Design review of the part built by this model. Coordinates are the model's own, in mm. A direction names the side the tool comes from. Coordinates: 2 decimals unless noted, no trailing zeros. Loops run counter-clockwise (first coordinate to the right, second up) from the corner with the lowest first, then second, coordinate; pieces in that order, holes last. Notation, with made-up numbers: M -29,65.5 L -8,65.5 A15 ccw -8,79.5 Z; hole C 84,85 d11. An arc over 180 degrees is marked long. Answer as a JSON object with one key per item and string values. Group by question number.
1. Consider section A-A (z = 8.5). Count the separate pieces of the cut face and the enclosed holes in it, then the cut area to 3 significant figures.
2. Draft analysis for pull direction Y (two halves, no side actions). For faces 1 (the flat face through (-1, 0, 7)), 2 (the cylindrical face through (36.41, -58.99, 6.9)), 3 (the cylindrical face through (58.975, -52.273, 6.902)), 4 (the flat face through (125, -35, 7)), state which applies: +Y half, -Y half, draft (parallel to the pull), parting line (faces both ways), or undercut.
3. Consider section C-C (x = -22.5). State the section outline as (y, z) points, then the cut area to 3 significant figures.
4. Insertion check: pin 1 (7 mm diameter, centred on x = 34.33, y = -55, fed in from +Z); pin 2 (4 mm diameter, centred on x = -18, z = 5.5, fed in from +Y). Each pin has a flat end and moves straight along its axis. Give the tip position at first contact, or say it passes through.
5. Machinability: for faces 5 (the flat face through (-110, 0, 7)), 6 (the flat face through (-2, -27, 0)), 7 (the flat face through (110, 0, 7)), which of the approach directions +Z, -Z, +X, -X, +Y, -Y give a long, thin tool a straight path to every point of the face, cutting with its end or side? Answer none if there is none.
6. Consider section B-B (x = -97.5). State the section outline as (y, z) points.
7. To check wall thickness, follow probe 1 along Y at (x, z) = (46, 8.75); probe 2 along Y at (x, z) = (12.5, 8.5); probe 3 along X at (y, z) = (-57.5, 3) (3 decimals). State the ranges of each line that lie inside material, in increasing order.
from build123d import *

# Parameters (mm, degrees)
F0_W     = 250
F0_H     = 70
F0_R     = 1.75
F0_R_2   = 5.75
F0_R_3   = 4.5
F0_R_4   = 3.5
F0_R_5   = 2.75
F0_R_6   = 2.25
F0_R_7   = 1.5
F0_R_8   = 1.25
F0_R_9   = 1
F0_R_10  = 3.75
F0_R_11  = 3.25
F0_R_12  = 3
F0_R_13  = 2.5
F0_R_14  = 2
F1_DEPTH = 14
F2_W     = 50
F2_H     = 14
F3_DEPTH = 14


with BuildPart() as f1:
    # F0 (on Top) → F1 (new body)
    with BuildSketch(Plane.XY):
        with Locations((0, -35)):
            Rectangle(F0_W, F0_H)
        with Locations((-89.333333, -55)):
            Circle(F0_R, mode=Mode.SUBTRACT)
        with Locations((-59.333333, -55)):
            Circle(F0_R, mode=Mode.SUBTRACT)
        with Locations((-29.333333, -55)):
            Circle(F0_R, mode=Mode.SUBTRACT)
        with Locations((16.333333, -55)):
            Circle(F0_R_2, mode=Mode.SUBTRACT)
        with Locations((34.333333, -55)):
            Circle(F0_R_3, mode=Mode.SUBTRACT)
        with Locations((48.333333, -55)):
            Circle(F0_R_4, mode=Mode.SUBTRACT)
        with Locations((59.333333, -55)):
            Circle(F0_R_5, mode=Mode.SUBTRACT)
        with Locations((68.333333, -55)):
            Circle(F0_R_6, mode=Mode.SUBTRACT)
        with Locations((76.333333, -55)):
            Circle(F0_R, mode=Mode.SUBTRACT)
        with Locations((84.333333, -55)):
            Circle(F0_R_7, mode=Mode.SUBTRACT)
        with Locations((92.333333, -55)):
            Circle(F0_R_8, mode=Mode.SUBTRACT)
        with Locations((100.333333, -55)):
            Circle(F0_R_9, mode=Mode.SUBTRACT)
        with Locations((-97.5, -20)):
            Circle(F0_R_10, mode=Mode.SUBTRACT)
        with Locations((-60, -20)):
            Circle(F0_R_11, mode=Mode.SUBTRACT)
        with Locations((-22.5, -20)):
            Circle(F0_R_12, mode=Mode.SUBTRACT)
        with Locations((12.5, -20)):
            Circle(F0_R_13, mode=Mode.SUBTRACT)
        with Locations((45, -20)):
            Circle(F0_R_6, mode=Mode.SUBTRACT)
        with Locations((75, -20)):
            Circle(F0_R_14, mode=Mode.SUBTRACT)
        with Locations((105, -20)):
            Circle(F0_R, mode=Mode.SUBTRACT)
    extrude(amount=F1_DEPTH)

    # F2 (on face) → F3 (join)
    with BuildSketch(Plane(origin=(0, 0, 0), x_dir=(-1, 0, 0), z_dir=(0, 1, 0))):
        with Locations((70, 7)):
            Rectangle(F2_W, F2_H)
        with Locations((-70, 7)):
            Rectangle(F2_W, F2_H)
    extrude(amount=F3_DEPTH)


solid = f1.part
Findings below:
{
 "1": {"separate pieces": "1", "enclosed holes": "19", "area": "18,400 mm^2"},
 "2": {"face 1": "+Y half", "face 2": "undercut", "face 3": "undercut", "face 4": "draft"},
 "3": {"outline": "M -70,0 L -23,0 L -23,14 L -70,14 Z; M -17,0 L 0,0 L 0,14 L -17,14 Z", "area": "896 mm^2"},
 "4": {"pin 1": "passes through", "pin 2": "stops at y = 0"},
 "5": {"face 5": "+Z, -Z, -X, +Y", "face 6": "-Z, +X, -X, +Y, -Y", "face 7": "+Z, -Z, +X, +Y"},
 "6": {"outline": "M -70,0 L -23.75,0 L -23.75,14 L -70,14 Z; M -16.25,0 L 0,0 L 0,14 L -16.25,14 Z"},
 "7": {"probe 1": "y = -70 to -57.61, -52.39 to -22.02, -17.98 to 14", "probe 2": "y = -70 to -59.29, -50.71 to -22.5, -17.5 to 0", "probe 3": "x = -125 to 11.155, 21.511 to 30.592, 38.075 to 45.884, 50.783 to 58.188, 60.479 to 125"}
}
